Verification items for the finished model (mm, model axes). Face numbers are marked on the shaded views. A direction names the side the tool comes from. Give positions to 0.01 mm unless a question says otherwise; leave off trailing zeros. Write each loop counter-clockwise with the first axis right and the second up, starting at its lowest first coordinate (ties: lowest second). Pieces come first, ordered by that corner, then holes. Notation, with made-up numbers: (65, -25.5) - (116, -25.5) arc R25 cw to (116, 13.5) - close; hole circle Ø10 at (28.25, 21). An arc over 180 degrees is marked (long way). Put each result on its own line as item: value.
from build123d import *

# Parameters (mm, degrees)
EXTRUDE_1_DEPTH     = 28.96
SKETCH_2_R          = 1.525
CUT_EXTRUDE_1_DEPTH = 3


with BuildPart() as part:
    # 草图1 → 凸台-拉伸1 (new body)
    with BuildSketch(Plane.XY):
        Polygon((-10, 8), (10, 8), (10, 0), (4.5, 0), (4.5, 4.5), (-4.5, 4.5), (-4.5, 0), (-10, 0), align=None)
    extrude(amount=EXTRUDE_1_DEPTH)

    # 草图2 → 切除-拉伸1 (cut)
    with BuildSketch(Plane(origin=(0, 8, 0), x_dir=(1, 0, 0), z_dir=(0, 1, 0))):
        with Locations(Location((7.5, -9.48, 0), (0, 0, 180))):
            Circle(SKETCH_2_R)
        with Locations((7.5, -19.48)):
            Circle(SKETCH_2_R)
        with Locations(Location((-7.5, -19.48, 0), (0, 0, 180))):
            Circle(SKETCH_2_R)
        with Locations((-7.5, -9.48)):
            Circle(SKETCH_2_R)
    extrude(amount=-CUT_EXTRUDE_1_DEPTH, mode=Mode.SUBTRACT)


solid = part.part
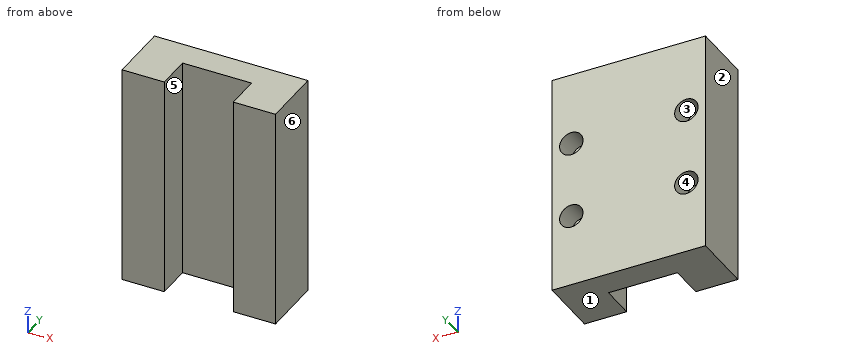
Q1. Section check A-A, the plane y = 0.5. Record the cut outline in (x, z), plus the area to 3 significant figures.
Answers follow:
outline: (-10, 0) - (-4.5, 0) - (-4.5, 28.96) - (-10, 28.96) - close; (4.5, 0) - (10, 0) - (10, 28.96) - (4.5, 28.96) - close
area: 319 mm2
Q2. Section check D-D, the plane x = 7.5. Record the cut outline in (y, z) (3 decimals), plus the area to 3 significant figures.
Answers follow:
outline: (0, 0) - (8, 0) - (8, 7.955) - (5, 7.955) - (5, 11.005) - (8, 11.005) - (8, 17.955) - (5, 17.955) - (5, 21.005) - (8, 21.005) - (8, 28.96) - (0, 28.96) - close
area: 213 mm2
Q3. Section check C-C, the plane y = 6.5. Record the cut outline in (x, z) (3 decimals), plus the area to 3 significant figures.
Answers follow:
outline: (-10, 0) - (10, 0) - (10, 28.96) - (-10, 28.96) - close; hole circle Ø3.05 at (-7.5, 9.48); hole circle Ø3.05 at (-7.5, 19.48); hole circle Ø3.05 at (7.5, 9.48); hole circle Ø3.05 at (7.5, 19.48)
area: 550 mm2
Q4. Scan lines: line 1 along Z through (x, y) = (-7.5, 6.4) (3 decimals); line 2 along X through (y, z) = (3, 7.5); line 3 along X through (y, z) = (7, 9). Record each from-to range of solid material in increasing order.
Answers follow:
line 1: z = 0 to 7.955, 11.005 to 17.955, 21.005 to 28.96
line 2: x = -10 to -4.5, 4.5 to 10
line 3: x = -10 to -8.95, -6.05 to 6.05, 8.95 to 10
Q5. Go/stop test with flat-tipped pins: pin 1 Ø2.5 at (x, z) = (-1.5, 12.5) entering from -Y; pin 2 Ø2.5 at (x, z) = (7.5, 19.48) entering from +Y. Record where each tip stops, or that it passes through.
Answers follow:
pin 1: stops at y = 4.5
pin 2: stops at y = 5
Q6. Release check for a two-part mould opening along Z. For the marked faces 1, 2 and 3 record: released by +Z, released by -Z, zero draft, split by the parting line, or undercut.
Answers follow:
face 1: released by -Z
face 2: zero draft
face 3: undercut
Q7. Set-up check for the marked faces 4, 5 and 6: record each of +Z, -Z, +X, -X, +Y, -Y from which the full face is reachable in a straight line by a thin tool's end or side.
Answers follow:
face 4: +Y
face 5: +Z, -Z, -Y
face 6: +Z, -Z, +X, +Y, -Y
Q8. Section check B-B, the plane z = 19.48. Record the cut outline in (x, y) (3 decimals).
Answers follow:
outline: (-10, 0) - (-4.5, 0) - (-4.5, 4.5) - (4.5, 4.5) - (4.5, 0) - (10, 0) - (10, 8) - (9.025, 8) - (9.025, 5) - (5.975, 5) - (5.975, 8) - (-5.975, 8) - (-5.975, 5) - (-9.025, 5) - (-9.025, 8) - (-10, 8) - close
